```python
from build123d import *

# Parameters (mm, degrees)
SKETCH1_W           = 120.8024
SKETCH1_H           = 83.9724
BOSS_EXTRUDE1_DEPTH = 5.7912
SKETCH2_W           = 40.267466666
SKETCH2_H           = 5.7912
CUT_EXTRUDE1_DEPTH  = 74.788101679
SKETCH9_W           = 5.7912
SKETCH9_H           = 27.9908
CUT_EXTRUDE8_DEPTH  = 74.788101679
CAVITY1_START       = -41.9862
CAVITY1_OUTLINE_W   = 40.267466667
CAVITY1_OUTLINE_H   = 5.7912
CAVITY1_DEPTH       = 5.7912
CAVITY1_START_2     = 13.9954
CAVITY1_2_OUTLINE_W = 5.7912
CAVITY1_2_OUTLINE_H = 5.7912
CAVITY1_2_DEPTH     = 27.9908
CAVITY1_START_3     = -36.195
CAVITY1_3_OUTLINE_W = 5.7912
CAVITY1_3_OUTLINE_H = 5.7912
CAVITY1_3_DEPTH     = 22.1996
SKETCH12_R          = 5.8674
SKETCH12_W          = 10.922
SKETCH12_H          = 12.7
CUT_EXTRUDE11_DEPTH = 74.788101679


# Read off the part's stored shape, not the designer's step: Cavity1
with BuildPart() as part:
    # Sketch1 → Boss-Extrude1 (new body)
    with BuildSketch(Plane.XY):
        Rectangle(SKETCH1_W, SKETCH1_H)
    extrude(amount=BOSS_EXTRUDE1_DEPTH)

    # Sketch2 → Cut-Extrude1 (cut, through all)
    with BuildSketch(Plane.XY.offset(5.7912)):
        with Locations((0, 39.0906)):
            Rectangle(SKETCH2_W, SKETCH2_H)
    extrude(amount=-CUT_EXTRUDE1_DEPTH, mode=Mode.SUBTRACT)

    # Sketch9 → Cut-Extrude8 (cut, through all)
    with BuildSketch(Plane.XY.offset(5.7912)):
        with Locations((-57.5056, 0)):
            Rectangle(SKETCH9_W, SKETCH9_H)
    extrude(amount=-CUT_EXTRUDE8_DEPTH, mode=Mode.SUBTRACT)

    # Cavity1 outline → Cavity1 (cut)
    with BuildSketch(Plane(origin=(0, 0, 0), x_dir=(1, 0, 0), z_dir=(0, 1, 0)).offset(CAVITY1_START)):
        with Locations((40.267466666, -2.8956)):
            Rectangle(CAVITY1_OUTLINE_W, CAVITY1_OUTLINE_H)
        with Locations((-40.267466666, -2.8956)):
            Rectangle(CAVITY1_OUTLINE_W, CAVITY1_OUTLINE_H)
    extrude(amount=CAVITY1_DEPTH, mode=Mode.SUBTRACT)

    # Cavity1 2 outline → Cavity1 2 (cut)
    with BuildSketch(Plane(origin=(0, 0, 0), x_dir=(1, 0, 0), z_dir=(0, 1, 0)).offset(CAVITY1_START_2)):
        with Locations((57.5056, -2.8956)):
            Rectangle(CAVITY1_2_OUTLINE_W, CAVITY1_2_OUTLINE_H)
    extrude(amount=CAVITY1_2_DEPTH, mode=Mode.SUBTRACT)

    # Cavity1 3 outline → Cavity1 3 (cut)
    with BuildSketch(Plane(origin=(0, 0, 0), x_dir=(1, 0, 0), z_dir=(0, 1, 0)).offset(CAVITY1_START_3)):
        with Locations((57.5056, -2.8956)):
            Rectangle(CAVITY1_3_OUTLINE_W, CAVITY1_3_OUTLINE_H)
    extrude(amount=CAVITY1_3_DEPTH, mode=Mode.SUBTRACT)

    # Sketch12 → Cut-Extrude11 (cut, through all)
    with BuildSketch(Plane.XY.offset(5.7912)):
        with Locations((-45.095282218, 28.294994395)):
            Circle(SKETCH12_R)
        with Locations((0, 28.294994395)):
            Circle(SKETCH12_R)
        with Locations((-777.151378692, 665.228044766)):
            Rectangle(SKETCH12_W, SKETCH12_H)
        with BuildLine():
            Line((43.470269973, 31.538321778), (43.470269973, 25.051667013))
            ThreePointArc((43.470269973, 25.051667013), (32.713369973, 28.294994395), (43.470269973, 31.538321778))
        make_face()
    extrude(amount=-CUT_EXTRUDE11_DEPTH, mode=Mode.SUBTRACT)


solid = part.part
```
Verification items for the finished model (mm, model axes). A direction names the side the tool comes from. Coordinates: 2 decimals unless noted, no trailing zeros. Write each loop counter-clockwise with the first axis right and the second up, starting at its lowest first coordinate (ties: lowest second). Pieces come first, ordered by that corner, then holes. Notation, with made-up numbers: (-27, 33.25) - (-11, 33.25) arc R9 ccw to (-11, 40.25) - close; hole circle Ø6 at (86.25, 44). An arc over 180 degrees is marked (long way). Write item = value, one per line.
Q1. Cross-section at A-A (x = 0). Enter the section's corners in (y, z) (3 decimals).
Answer:
outline = (-41.986, 0) - (22.428, 0) - (22.428, 5.791) - (-41.986, 5.791) - close; (34.162, 0) - (36.195, 0) - (36.195, 5.791) - (34.162, 5.791) - close
Q2. Cross-section at C-C (y = 9). Enter the section's corners in (x, z), plus the area to 3 significant figures.
Answer:
outline = (-54.61, 0) - (60.4, 0) - (60.4, 5.79) - (-54.61, 5.79) - close
area = 666 mm²
Q3. Material ranges on L1, parallel to Y at x = 0, z = 2.25 (3 decimals); L2, parallel to X at y = -3.5, z = 4.15; L3, parallel to Y at x = 31.5, z = 3.05 (3 decimals), recorded low to high. Write a range as from..to.
Answer:
L1 = -41.986..22.428, 34.162..36.195
L2 = -54.61..60.4
L3 = -36.195..41.986
Q4. Access from +Z, -Z, +X, -X, +Y, -Y to the whole of each face (thin tool, end or side, straight path). Record for faces 4 (the face through (20.134, 39, 3)), 5 (the face through (-54.61, 0, 3)), 6 (the face through (-41, -36.195, 3)), 7 (the face through (57, 13.995, 3)), 8 (the face through (20.134, -39, 3)).
Answer:
face_4 = +Z, -Z, +Y
face_5 = +Z, -Z, -X
face_6 = +Z, -Z, -X, -Y
face_7 = +Z, -Z, +X, +Y
face_8 = +Z, -Z, +X, -Y
Q5. Go/stop test with flat-tipped pins: pin 1 Ø3 at (y, z) = (-27.5, 3.5) entering from +X; pin 2 Ø7 at (x, y) = (0, 28.29) entering from +Z; pin 3 Ø1.7 at (x, z) = (7.5, 1.5) entering from +Y (3 decimals); pin 4 Ø3 at (x, z) = (-42, 2.5) entering from -Y (3 decimals). Record where each tip stops, or that it passes through.
Answer:
pin_1 = 54.61
pin_2 = through
pin_3 = 36.195
pin_4 = -36.195
Q6. Cross-section at B-B (z = 1.05). Enter the section's corners in (x, y) (3 decimals), plus the area to 3 significant figures.
Answer:
outline = (-60.401, -36.195) - (-20.134, -36.195) - (-20.134, -41.986) - (20.134, -41.986) - (20.134, -36.195) - (54.61, -36.195) - (54.61, -13.995) - (60.401, -13.995) - (60.401, 13.995) - (54.61, 13.995) - (54.61, 41.986) - (20.134, 41.986) - (20.134, 36.195) - (-20.134, 36.195) - (-20.134, 41.986) - (-60.401, 41.986) - (-60.401, 13.995) - (-54.61, 13.995) - (-54.61, -13.995) - (-60.401, -13.995) - close; hole circle Ø11.735 at (-45.095, 28.295); hole circle Ø11.735 at (0, 28.295); hole (43.47, 25.052) - (43.47, 31.538) arc R5.867 ccw (long way) to start
area = 8,670 mm²
Q7. Cross-section at D-D (x = 16). Enter the section's corners in (y, z) (3 decimals).
Answer:
outline = (-41.986, 0) - (36.195, 0) - (36.195, 5.791) - (-41.986, 5.791) - close
Q8. Mould release check, pull along Y, two halves, no side actions. Record for faces 1 (the face through (60.401, 0, 3)), 2 (the face through (37, -36.195, 3)), 3 (the face through (-45.859, 34.112, 2.936)): released by +Y, released by -Y, zero draft, split by the parting line, or undercut.
Answer:
face_1 = zero draft
face_2 = released by -Y
face_3 = undercut
